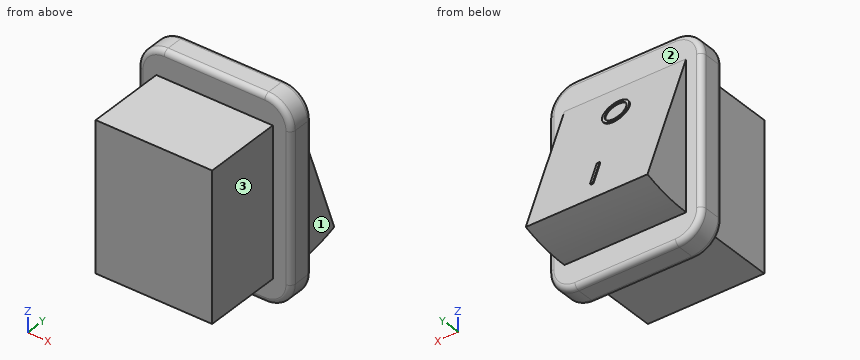
from build123d import *

# Parameters (mm, degrees)
SKETCH_1_W      = 22
SKETCH_1_H      = 28
EXTRUDE_2_DEPTH = 15
SKETCH_1_5_W    = 29
SKETCH_1_5_H    = 38
SKETCH_1_5_W_2  = 22
SKETCH_1_5_H_2  = 28
EXTRUDE_3_DEPTH = 5
SKETCH_2_W      = 23
SKETCH_2_H      = 28
REVOLVE_1_ANGLE = 20
SKETCH_3_R      = 2.5
SKETCH_3_R_2    = 2
SKETCH_3_W      = 0.5
SKETCH_3_H      = 5
EXTRUDE_4_DEPTH = 0.2
FILLET_1_R      = 5
FILLET_2_R      = 1


with BuildPart() as part:
    # Sketch 1 → Extrude 2 (new body)
    with BuildSketch(Plane(origin=(0, 0, 0), x_dir=(1, 0, 0), z_dir=(0, 1, 0))):
        Rectangle(SKETCH_1_W, SKETCH_1_H)
    extrude(amount=-EXTRUDE_2_DEPTH)

    # Sketch 1_5 → Extrude 3 (add)
    # profile 1 of 2: a face of its own
    with BuildSketch(Plane(origin=(0, 0, 0), x_dir=(1, 0, 0), z_dir=(0, 1, 0))):
        Rectangle(SKETCH_1_5_W, SKETCH_1_5_H)
        Rectangle(SKETCH_1_5_W_2, SKETCH_1_5_H_2, mode=Mode.SUBTRACT)
    # profile 2 of 2: a face of its own
    with BuildSketch(Plane(origin=(0, 0, 0), x_dir=(1, 0, 0), z_dir=(0, 1, 0))):
        Rectangle(SKETCH_1_5_W_2, SKETCH_1_5_H_2)
    extrude(amount=EXTRUDE_3_DEPTH)

    # Sketch 2 → Revolve 1 (revolve)
    with BuildSketch(Plane(origin=(0, 5, 0), x_dir=(1, 0, 0), z_dir=(0, 1, 0))):
        Rectangle(SKETCH_2_W, SKETCH_2_H)
    revolve(axis=Axis((-11.5, 5, 14), (1, 0, 0)), revolution_arc=REVOLVE_1_ANGLE)

    # Sketch 3 → Extrude 4 (add)
    # profile 1 of 2: a face of its own
    with BuildSketch(Plane(origin=(0, 8.914624376, 3.244657922), x_dir=(1, 0, 0), z_dir=(0, 0.9396926207859082, 0.34202014332566943))):
        with Locations(Location((0, -4.945595974, 0), (0, 0, 270))):
            Circle(SKETCH_3_R)
        with Locations(Location((0, -4.945595974, 0), (0, 0, 270))):
            Circle(SKETCH_3_R_2, mode=Mode.SUBTRACT)
    # profile 2 of 2: a face of its own
    with BuildSketch(Plane(origin=(0, 8.914624376, 3.244657922), x_dir=(1, 0, 0), z_dir=(0, 0.9396926207859082, 0.34202014332566943))):
        with Locations((0, 10.054404026)):
            Rectangle(SKETCH_3_W, SKETCH_3_H)
    extrude(amount=EXTRUDE_4_DEPTH)

    # Fillet 1
    fillet_1_edges = [part.edges().sort_by_distance(p)[0] for p in [
        (-14.5, 2.5, -19),
        (-14.5, 2.5, 19),
        (14.5, 2.5, 19),
        (14.5, 2.5, -19),
    ]]
    fillet(fillet_1_edges, radius=FILLET_1_R)

    # Fillet 2
    fillet_2_edges = [part.edges().sort_by_distance(p)[0] for p in [
        (-14.5, 0, 0),
        (-14.5, 5, 0),
        (0, 0, -19),
        (14.5, 0, 0),
        (0, 0, 19),
        (-13.035533906, 0, 17.535533906),
        (13.035533906, 0, 17.535533906),
        (13.035533906, 0, -17.535533906),
        (-13.035533906, 0, -17.535533906),
        (0, 5, -19),
        (0, 5, 19),
        (14.5, 5, 0),
        (-13.035533906, 5, 17.535533906),
        (13.035533906, 5, 17.535533906),
        (13.035533906, 5, -17.535533906),
        (-13.035533906, 5, -17.535533906),
    ]]
    fillet(fillet_2_edges, radius=FILLET_2_R)


solid = part.part
Input: part model. Units: mm. Frame: model coordinates. Face numbers are marked on the shaded views. A direction names the side the tool comes from. Coordinates: 2 decimals unless noted, no trailing zeros. Loops run counter-clockwise (first coordinate to the right, second up) from the corner with the lowest first, then second, coordinate; pieces in that order, holes last.
Q1. Set-up query: the marked faces 1, 2 and 3. Return all of +Z, -Z, +X, -X, +Y, -Y with unobstructed straight access to the full face (end or side cutting, diameter ignored); none if empty.
Q2. Material intervals for line 1 (X direction, y = -2.25, z = -9.5); line 2 (Y direction, x = 11.75, z = -0.5); line 3 (Z direction, x = 12.5, y = 2.25), sorted ascending.
Q3. Cut plane C-C (y = -7.5). Output: boundary loops of the cut face in (x, z), then the cut area to 3 significant figures.
Q4. Contact query for flat-ended pins moving along their axis: pin 1 (5 mm diameter, centred on y = -11.5, z = 11.5, fed in from -X); pin 2 (5 mm diameter, centred on y = -7.5, z = -2.5, fed in from +X); pin 3 (3 mm diameter, centred on y = 11.5, z = 2.5, fed in from -X); pin 4 (3 mm diameter, centred on x = -9.5, y = 7, fed in from -Z). Output: stop coordinate, or through.
Q5. Cut plane A-A (x = -3.75). Output: boundary loops of the cut face in (y, z), then the cut area to 3 significant figures.
Q6. Cut plane B-B (z = -9.5). Output: boundary loops of the cut face in (x, y), then the cut area to 3 significant figures.
Q7. Cut plane D-D (z = 0). Output: boundary loops of the cut face in (x, y), then the cut area to 3 significant figures.
Working result:
1. face 1: +Z, -Z, +X, +Y
1. face 2: +Y
1. face 3: +Z, -Z, +X, -Y
2. line 1: x = -11 to 11
2. line 2: y = 0 to 5
2. line 3: z = -18 to 18
3. outline: (-11, -14) - (11, -14) - (11, 14) - (-11, 14) - close
3. area: 616 mm2
4. pin 1: stops at x = -11
4. pin 2: stops at x = 11
4. pin 3: passes through
4. pin 4: stops at z = -14
5. outline: (-15, -14) - (0, -14) - (0, -18) arc R1 ccw to (1, -19) - (4, -19) arc R1 ccw to (5, -18) - (5, -14) arc R28 ccw to (14.58, -12.31) - (5, 14) - (5, 18) arc R1 ccw to (4, 19) - (1, 19) arc R1 ccw to (0, 18) - (0, 14) - (-15, 14) - close
5. area: 746 mm2
6. outline: (-14.5, 1) arc R1 ccw to (-13.5, 0) - (-11, 0) - (-11, -15) - (11, -15) - (11, 0) - (13.5, 0) arc R1 ccw to (14.5, 1) - (14.5, 4) arc R1 ccw to (13.5, 5) - (11.5, 5) - (11.5, 13.55) - (-11.5, 13.55) - (-11.5, 5) - (-13.5, 5) arc R1 ccw to (-14.5, 4) - close
6. area: 671 mm2
7. outline: (-14.5, 1) arc R1 ccw to (-13.5, 0) - (-11, 0) - (-11, -15) - (11, -15) - (11, 0) - (13.5, 0) arc R1 ccw to (14.5, 1) - (14.5, 4) arc R1 ccw to (13.5, 5) - (11.5, 5) - (11.5, 10.1) - (-11.5, 10.1) - (-11.5, 5) - (-13.5, 5) arc R1 ccw to (-14.5, 4) - close
7. area: 591 mm2
